Build history of the part. All positions in model axes, mm. Face numbers are marked on the shaded views. A direction names the side the tool comes from. Give positions to 0.01 mm unless a question says otherwise; leave off trailing zeros. Loops run counter-clockwise (first coordinate to the right, second up) from the corner with the lowest first, then second, coordinate; pieces in that order, holes last. Notation, with made-up numbers: (-39, 30) -> (13, 30) arc R21 cw to (13, 51) -> close; hole circle Ø1 at (-28.5, 15.25). An arc over 180 degrees is marked (long way). Answer as a JSON object with one key per item and string values. Group by question number.
Q1. Tool access for the marked faces 4, 5, 6 and 7: list every direction of +Z, -Z, +X, -X, +Y, -Y with a clear straight run to the whole face (end or side of a thin tool).
Q2. Wall check: probe 1 along X at (y, z) = (5.3, -11.95); probe 2 along X at (y, z) = (3, -4.5); probe 3 along Z at (x, y) = (8, 7.25). Give the ranges that are in metal, low to high. Write a range as from..to.
Q3. Band-saw the part on B-B, the plane x = -2.25. Write the cut outline in (y, z), plus the area to 3 significant figures.
Q4. Drop flat-ended pins along their axis: pin 1 (2 mm diameter, centred on x = 7.5, z = -11.95, fed in from +Y); pin 2 (3 mm diameter, centred on x = -7.5, z = -27.95, fed in from +Y); pin 3 (2 mm diameter, centred on x = 0.5, z = -7, fed in from +Y). Give the stop position or say it passes through.
Q5. Two-plate mould, pull along X, no slides. Class the marked faces 1, 2 and 3: pulls with the +X half, pulls with the -X half, needs draft (parallel to the pull), parting line crosses it, or undercut.
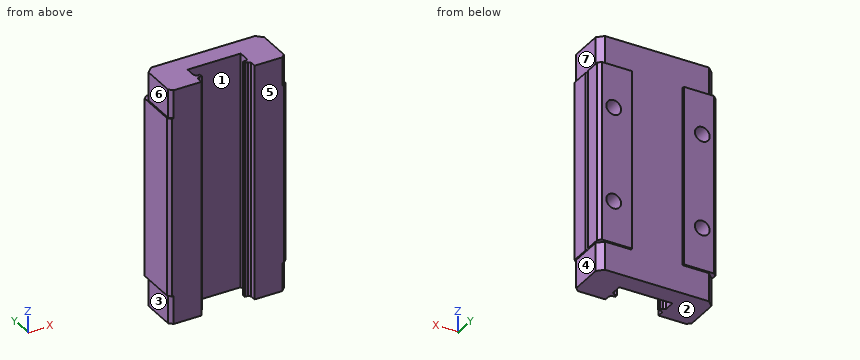
from build123d import *

# Parameters (mm, degrees)
EXTRUDE_1_DEPTH     = 39.9
CHAMFER_1_SIZE      = 0.5
CUT_EXTRUDE_1_DEPTH = 0.3
SKETCH_6_W          = 0.2
SKETCH_6_H          = 4.8
CUT_EXTRUDE_2_DEPTH = 8.3
CHAMFER_2_SIZE      = 1
CHAMFER_3_SIZE      = 0.6
CHAMFER_4_SIZE      = 0.5
SKETCH_7_R          = 0.4
CUT_EXTRUDE_3_DEPTH = 30.3


with BuildPart() as part:
    # 草图1 → 凸台-拉伸1 (new body)
    with BuildSketch(Plane.XY):
        Polygon((-10, 0), (-10, 7.5), (10, 7.5), (10, 0), (4.5, 0), (4.5, 1), (4.146446609, 1.353553391), (3.646446609, 1.353553391), (3.646446609, 1.853553391), (4.146446609, 1.853553391), (4.5, 2.207106781), (4.5, 4), (-4.5, 4), (-4.5, 2.207106781), (-4.146446609, 1.853553391), (-3.646446609, 1.853553391), (-3.646446609, 1.353553391), (-4.146446609, 1.353553391), (-4.5, 1), (-4.5, 0), align=None)
    extrude(amount=-EXTRUDE_1_DEPTH)

    # 草图3 → M3 螺纹孔1 (revolve, cut)
    with BuildSketch(Plane(origin=(7.5, 7.5, -27.95), x_dir=(0, 0, 1), z_dir=(1, 0, 0))):
        Polygon((0, 0), (0, 3.751075774), (1.25, 3), (1.25, 0), align=None)
    hole_wizard_m3_1 = revolve(axis=Axis((7.5, 13.85, -27.95), (0, -1, 0)), mode=Mode.SUBTRACT)

    # 镜向1: M3 螺纹孔1 across plane
    add(hole_wizard_m3_1.mirror(Plane(origin=(0, 0, -19.95), x_dir=(1, 0, 0), z_dir=(0, 0, -1))), mode=Mode.SUBTRACT)

    # 镜向2: M3 螺纹孔1 across plane
    add(hole_wizard_m3_1.mirror(Plane.ZY), mode=Mode.SUBTRACT)

    # 镜向2 copy 1 sketch → 镜向2 copy 1 (revolve, cut)
    with BuildSketch(Plane(origin=(-7.5, 7.5, -11.95), x_dir=(0, 0, -1), z_dir=(-1, 0, 0))):
        Polygon((0, 0), (0, 3.751075774), (1.25, 3), (1.25, 0), align=None)
    revolve(axis=Axis((-7.5, 13.85, -11.95), (0, -1, 0)), mode=Mode.SUBTRACT)

    # 倒角1
    chamfer_1_edges = [part.edges().sort_by_distance(p)[0] for p in [
        (10, 7.5, -19.95),
        (-10, 7.5, -19.95),
    ]]
    chamfer(chamfer_1_edges, length=CHAMFER_1_SIZE)

    # 草图5 → 切除-拉伸1 (cut)
    with BuildSketch(Plane(origin=(0, 7.5, 0), x_dir=(1, 0, 0), z_dir=(0, 1, 0))):
        Polygon((-9.5, 35.1), (-4.368581018, 35.1), (-4.368581018, 4.8), (-9.5, 4.8), (-10, 4.8), (-10, 0), (10, 0), (10, 4.8), (9.5, 4.8), (4.368581018, 4.8), (4.368581018, 35.1), (9.5, 35.1), (10, 35.1), (10, 39.9), (-10, 39.9), (-10, 35.1), align=None)
    extrude(amount=-CUT_EXTRUDE_1_DEPTH, mode=Mode.SUBTRACT)

    # 草图6 → 切除-拉伸2 (cut)
    with BuildSketch(Plane(origin=(0, 7.2, 0), x_dir=(1, 0, 0), z_dir=(0, 1, 0))):
        with Locations((-9.9, 37.5)):
            Rectangle(SKETCH_6_W, SKETCH_6_H)
        with Locations((9.9, 37.5)):
            Rectangle(SKETCH_6_W, SKETCH_6_H)
        with Locations((9.9, 2.4)):
            Rectangle(SKETCH_6_W, SKETCH_6_H)
        with Locations((-9.9, 2.4)):
            Rectangle(SKETCH_6_W, SKETCH_6_H)
    extrude(amount=-CUT_EXTRUDE_2_DEPTH, mode=Mode.SUBTRACT)

    # 倒角2
    # the kernel refuses this chamfer: 1 mm, written as the material it takes off along each edge
    with BuildSketch(Plane(origin=(-9.8, 7.2, -4.8), x_dir=(-0.027495876610583895, -0.9996219169112968, 0), z_dir=(0, 0, 1)), Plane(origin=(-9.8, 7.2, -42.471682988), x_dir=(-0.027495876610585623, -0.9996219169112968, 0), z_dir=(0, 0, 1))) as chamfer_2_piece_1:
        Polygon((CHAMFER_2_SIZE * 0.999621916911, CHAMFER_2_SIZE * 0.0274958766106), (-CHAMFER_2_SIZE * 0.0274958766106, CHAMFER_2_SIZE * 0.999621916911), (0, 0), align=None)
    extrude(amount=7.371682988, mode=Mode.SUBTRACT)
    with BuildSketch(Plane(origin=(9.8, 7.2, 2.571682988), x_dir=(-0.9996219169112968, 0.02749587661058651, 0), z_dir=(0, 0, -1)), Plane(origin=(9.8, 7.2, -35.1), x_dir=(-0.9996219169112968, 0.02749587661058651, 0), z_dir=(0, 0, -1))) as chamfer_2_piece_2:
        Polygon((CHAMFER_2_SIZE * 0.999621916911, -CHAMFER_2_SIZE * 0.0274958766106), (-CHAMFER_2_SIZE * 0.0274958766106, -CHAMFER_2_SIZE * 0.999621916911), (0, 0), align=None)
    extrude(amount=7.371682988, mode=Mode.SUBTRACT)

    # 倒角3
    chamfer_3_edges = [part.edges().sort_by_distance(p)[0] for p in [
        (-9.8, 0, -37.5),
        (9.8, 0, -37.5),
        (9.8, 0, -2.4),
        (-9.8, 0, -2.4),
    ]]
    chamfer(chamfer_3_edges, length=CHAMFER_3_SIZE)

    # 倒角4
    chamfer_4_edges = [part.edges().sort_by_distance(p)[0] for p in [
        (-10, 0, -19.95),
        (10, 0, -19.95),
    ]]
    chamfer(chamfer_4_edges, length=CHAMFER_4_SIZE)

    # 草图7 → 切除-拉伸3 (cut)
    with BuildSketch(Plane(origin=(0, 0, -35.1), x_dir=(-1, 0, 0), z_dir=(0, 0, -1))):
        with Locations((-10.2, 4)):
            Circle(SKETCH_7_R)
    extrude(amount=-CUT_EXTRUDE_3_DEPTH, mode=Mode.SUBTRACT)


solid = part.part
Worked answers:
{
 "1": {"face 4": "-Z, +X, +Y, -Y", "face 5": "+Z, -Z, +X, -X, -Y", "face 6": "+Z, -X, +Y, -Y", "face 7": "+Z, +X, +Y, -Y"},
 "2": {"probe 1": "-10..-8.75, -6.25..6.25, 8.75..10", "probe 2": "-9.8..-4.5, 4.5..9.8", "probe 3": "-35.1..-29.1, -26.8..-13.1, -10.8..-4.8"},
 "3": {"outline": "(4, -39.9) -> (7.2, -39.9) -> (7.2, 0) -> (4, 0) -> close", "area": "128 mm2"},
 "4": {"pin 1": "y = 4.35", "pin 2": "y = 7.5", "pin 3": "y = 7.2"},
 "5": {"face 1": "undercut", "face 2": "needs draft", "face 3": "pulls with the -X half"}
}
